Geometry check sheet. Reference: the model listing, model coordinates, mm. Face numbers are marked on the shaded views. Round coordinates to 2 decimals unless told otherwise and drop trailing zeros. Loops run counter-clockwise (first coordinate to the right, second up) from the corner with the lowest first, then second, coordinate; pieces in that order, holes last. Notation, with made-up numbers: M 56.5,-34 L 78.5,-34 A15 cw 78.5,-16 Z; hole C -18,18 d4. An arc over 180 degrees is marked long. Write item = value, one per line.
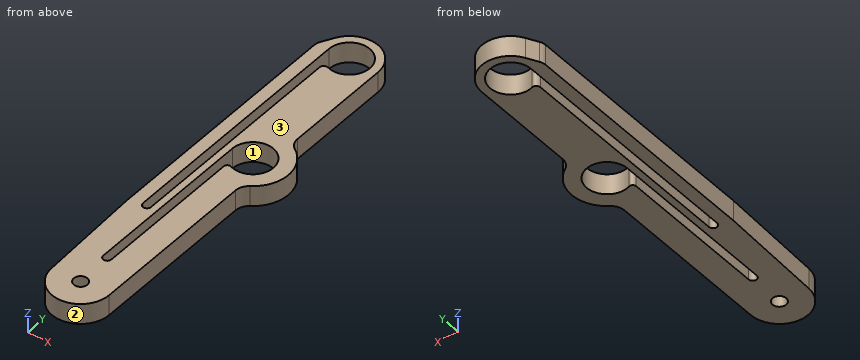
from build123d import *

# Parameters (mm, degrees)
SKETCH_1_R      = 1
EXTRUDE_1_DEPTH = 3


with BuildPart() as part:
    # 草图1 → 凸台-拉伸1 (new body)
    with BuildSketch(Plane.XY):
        with BuildLine():
            Line((-4.801725368, 51.134970407), (-4.801725368, 14.84551668))
            Line((-4.801725368, 14.84551668), (-4.196767432, -0.56475169))
            ThreePointArc((-4.196767432, -0.56475169), (0.0823917, -4.59919178), (4.2, -0.4))
            Line((4.2, -0.4), (4.2, 3))
            Line((4.2, 3), (4.2, 24.046707274))
            ThreePointArc((4.2, 24.046707274), (4.436165793, 24.989516316), (5.088888889, 25.709666113))
            ThreePointArc((5.088888889, 25.709666113), (7.4, 30.033359093), (5.088888889, 34.357052074))
            ThreePointArc((5.088888889, 34.357052074), (4.436165793, 35.077201871), (4.2, 36.020010912))
            Line((4.2, 36.020010912), (4.2, 47.4))
            Line((4.2, 47.4), (4.2, 51.6))
            ThreePointArc((4.2, 51.6), (1.019230191, 55.674453315), (-3.705318961, 53.577526587))
            Line((-3.705318961, 53.577526587), (-4.574814921, 52.00679382))
            ThreePointArc((-4.574814921, 52.00679382), (-4.743693388, 51.585307183), (-4.801725368, 51.134970407))
        make_face()
        with Locations((0, -0.4)):
            Circle(SKETCH_1_R, mode=Mode.SUBTRACT)
        with BuildLine():
            Line((-1.8, 15.6), (-1.8, 48.20588745))
            ThreePointArc((-1.8, 48.20588745), (-1.546410162, 48.695785399), (-1, 48.771572875))
            ThreePointArc((-1, 48.771572875), (2.449489743, 53.332050808), (-3, 51.6))
            Line((-3, 51.6), (-3, 15.6))
            ThreePointArc((-3, 15.6), (-2.4, 15), (-1.8, 15.6))
        make_face(mode=Mode.SUBTRACT)
        with BuildLine():
            Line((-0.8, 30.033359093), (-0.8, 5.033359093))
            ThreePointArc((-0.8, 5.033359093), (-0.2, 4.433359093), (0.4, 5.033359093))
            Line((0.4, 5.033359093), (0.4, 26.783743731))
            ThreePointArc((0.4, 26.783743731), (0.619694045, 27.197783067), (1.085714286, 27.247974497))
            ThreePointArc((1.085714286, 27.247974497), (4.684236014, 31.715194825), (-0.8, 30.033359093))
        make_face(mode=Mode.SUBTRACT)
    extrude(amount=EXTRUDE_1_DEPTH)


solid = part.part
(1) Sectioned sample at C-C on x = 2.5. Record the cut outline in (y, z).
Result set:
outline = M -3.77,0 L 27.05,0 L 27.05,3 L -3.77,3 Z; M 33.02,0 L 49.94,0 L 49.94,3 L 33.02,3 Z; M 53.26,0 L 54.97,0 L 54.97,3 L 53.26,3 Z
(2) Sectioned sample at A-A on y = 22. Record the cut outline in (x, z), then the cut area to 3 significant figures.
Result set:
outline = M -4.8,0 L -3,0 L -3,3 L -4.8,3 Z; M -1.8,0 L -0.8,0 L -0.8,3 L -1.8,3 Z; M 0.4,0 L 4.2,0 L 4.2,3 L 0.4,3 Z
area = 19.8 mm2
(3) Sectioned sample at D-D on y = 35.5. Record the cut outline in (x, z).
Result set:
outline = M -4.8,0 L -3,0 L -3,3 L -4.8,3 Z; M -1.8,0 L 4.27,0 L 4.27,3 L -1.8,3 Z
(4) Material ranges on line 1 along X through (y, z) = (25, 1.5); line 2 along X through (y, z) = (20, 1.65); line 3 along Y through (x, z) = (2.2, 1.8), recorded low to high. Write a range as from..to.
Result set:
line_1 = -4.8..-3, -1.8..-0.8, 0.4..4.44
line_2 = -4.8..-3, -1.8..-0.8, 0.4..4.2
line_3 = -3.98..27.03, 33.03..49.56, 53.64..55.18
(5) Depth check by flat-ended pin: pin 1 Ø1 at (x, y) = (5, 37) entering from -Z; pin 2 Ø3 at (x, y) = (0, -0.4) entering from +Z; pin 3 Ø0.9 at (y, z) = (38.5, 1.5) entering from +X. Enter the tip coordinate at first touch or a pass-through.
Result set:
pin_1 = through
pin_2 = 3
pin_3 = 4.2
(6) Release check for a two-part mould opening along Y. For the marked faces 1, 2 and 3 record: released by +Y, released by -Y, zero draft, split by the parting line, or undercut.
Result set:
face_1 = undercut
face_2 = released by -Y
face_3 = zero draft
(7) Sectioned sample at B-B on x = -0.2. Record the cut outline in (y, z).
Result set:
outline = M -4.6,0 L -1.38,0 L -1.38,3 L -4.6,3 Z; M 0.58,0 L 4.43,0 L 4.43,3 L 0.58,3 Z; M 31.83,0 L 48.61,0 L 48.61,3 L 31.83,3 Z; M 54.59,0 L 55.8,0 L 55.8,3 L 54.59,3 Z
